```python
from build123d import *

# Parameters (mm, degrees)
SKETCH007_R             = 1.65
PAD005_DEPTH            = 1.6
SKETCH008_R             = 3.55
PAD006_DEPTH            = 16.3
SKETCH009_R             = 1.95
POCKET002_DEPTH         = 12
POCKET003_DEPTH         = 1.6
BODY002_PLACEMENT_ANGLE = 180


with BuildPart() as part:
    # Sketch007 → Pad005 (new body)
    with BuildSketch(Plane.XY):
        with BuildLine():
            Line((-51.5, 40.5), (51.5, 40.5))
            ThreePointArc((54.5, 37.5), (53.62132, 39.62132), (51.5, 40.5))
            Line((54.5, 37.5), (54.5, 14))
            ThreePointArc((54.5, 14), (55.37868, 11.87868), (57.5, 11))
            Line((57.5, 11), (70.5, 11))
            ThreePointArc((73.5, 8), (72.62132, 10.12132), (70.5, 11))
            Line((73.5, 8), (73.5, 3))
            Line((73.5, 3), (75, 3))
            ThreePointArc((75, -3), (78, 0), (75, 3))
            Line((73.5, -3), (75, -3))
            Line((73.5, -3), (73.5, -8))
            ThreePointArc((70.5, -11), (72.62132, -10.12132), (73.5, -8))
            Line((70.5, -11), (57.5, -11))
            ThreePointArc((57.5, -11), (55.37868, -11.87868), (54.5, -14))
            Line((54.5, -14), (54.5, -37.5))
            ThreePointArc((51.5, -40.5), (53.62132, -39.62132), (54.5, -37.5))
            Line((51.5, -40.5), (-51.5, -40.5))
            ThreePointArc((-54.5, -37.5), (-53.62132, -39.62132), (-51.5, -40.5))
            Line((-54.5, -37.5), (-54.5, 37.5))
            ThreePointArc((-51.5, 40.5), (-53.62132, 39.62132), (-54.5, 37.5))
        make_face()
        with Locations((75, 0)):
            Circle(SKETCH007_R, mode=Mode.SUBTRACT)
    extrude(amount=PAD005_DEPTH)

    # Sketch008 → Pad006 (join)
    with BuildSketch(Plane.XY):
        with Locations((-49.75, 35.75)):
            Circle(SKETCH008_R)
        with Locations((-9.75, 35.75)):
            Circle(SKETCH008_R)
        with Locations((9.75, 35.75)):
            Circle(SKETCH008_R)
        with Locations((49.75, 35.75)):
            Circle(SKETCH008_R)
        with Locations((49.75, -35.75)):
            Circle(SKETCH008_R)
        with Locations((9.75, -35.75)):
            Circle(SKETCH008_R)
        with Locations((-9.75, -35.75)):
            Circle(SKETCH008_R)
        with Locations((-49.75, -35.75)):
            Circle(SKETCH008_R)
    extrude(amount=PAD006_DEPTH)

    # Sketch009 (on DatumPlane) → Pocket002 (cut)
    with BuildSketch(Plane.XY.offset(16.3)):
        with Locations((-49.75, 35.75)):
            Circle(SKETCH009_R)
        with Locations((-9.75, 35.75)):
            Circle(SKETCH009_R)
        with Locations((9.75, 35.75)):
            Circle(SKETCH009_R)
        with Locations((49.75, 35.75)):
            Circle(SKETCH009_R)
        with Locations((-49.75, -35.75)):
            Circle(SKETCH009_R)
        with Locations((-9.75, -35.75)):
            Circle(SKETCH009_R)
        with Locations((9.75, -35.75)):
            Circle(SKETCH009_R)
        with Locations((49.75, -35.75)):
            Circle(SKETCH009_R)
    extrude(amount=-POCKET002_DEPTH, mode=Mode.SUBTRACT)

    # Sketch011 → Pocket003 (cut)
    with BuildSketch(Plane.XY):
        with BuildLine():
            ThreePointArc((-25, 5), (-30, 0), (-25, -5))
            Line((-25, -5), (25, -5))
            ThreePointArc((25, -5), (30, 0), (25, 5))
            Line((25, 5), (-25, 5))
        make_face()
    extrude(amount=POCKET003_DEPTH, mode=Mode.SUBTRACT)


with BuildPart() as part_1:
    # Body002 placement: moved
    add(part.part.moved(Location((0, 0, 38))).rotate(Axis((0, 0, 38), (1, 0, 0)), BODY002_PLACEMENT_ANGLE))


solid = part_1.part
```
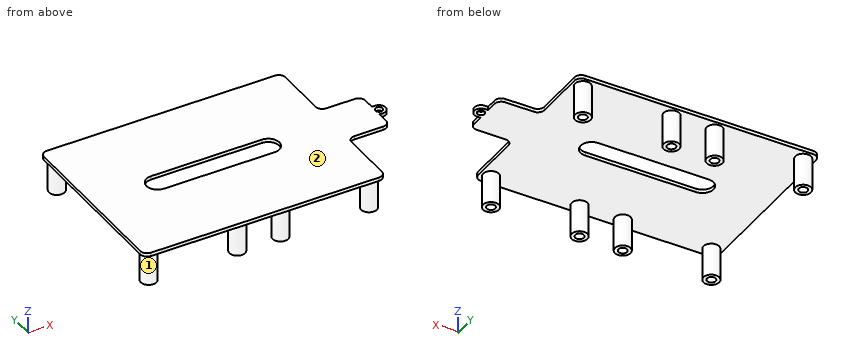
Part model, mm, in its own coordinate system. Face numbers are marked on the shaded views. Give positions to 0.01 mm unless a question says otherwise; leave off trailing zeros. Order: outer loops, then holes, each group sorted by start corner. A loop starts at its lowest first (then second) coordinate and runs counter-clockwise, first axis right, second up. Notation, with made-up numbers: M 35,-26 L 55,-26 A30 cw 55,4 Z; hole C -24,16.5 d4. An arc over 180 degrees is marked long. Use a Markdown table: item, result. Add a question column.
(1) Drop flat-ended pins along their axis: P1, Ø3, axis at x = -16, z = 33, coming from the +Y side; P2, Ø3.5, axis at x = -9.75, y = 35.75, coming from the -Z side; P3, Ø0.5, axis at y = 22.5, z = 37.5, coming from the +X side; P4, Ø1.5, axis at x = 38, y = 2.5, coming from the -Z side. Give the stop position or say it passes through.
(2) Mould opens along X. For the marked faces 1 and 2 say: +X half, -X half, draft (parallel to the pull), parting line (faces both ways), or undercut.
(3) Saw through at A-A, the plane z = 25.5. Give the number of separate pieces and of enclosed holes in the cut face, and give its area (3 significant figures).
(4) Probe line 1 along Y through (x, z) = (-49.75, 28.5); line 2 along X through (y, z) = (37, 36.25); line 3 along Z through (x, y) = (18, 16). List the from-to ranges inside material, lowest first. Write a range as [from, to].
(5) Saw through at C-C, the plane x = 49.75. Give the cut face in (y, z), and give its area (3 significant figures).
(6) Saw through at D-D, the plane y = 18.5. Give the cut face in (x, z).
(7) Saw through at B-B, the plane x = 20. Give the cut face in (y, z).
Answer key:
| question | item | result |
|---|---|---|
| 1 | P1 | through |
| 1 | P2 | z = 33.7 |
| 1 | P3 | x = 54.5 |
| 1 | P4 | z = 36.4 |
| 2 | face 1 | undercut |
| 2 | face 2 | draft |
| 3 | separate pieces | 8 |
| 3 | enclosed holes | 8 |
| 3 | area | 221 mm^2 |
| 4 | line 1 | [-39.3, -37.7], [-33.8, -32.2], [32.2, 33.8], [37.7, 39.3] |
| 4 | line 2 | [-53.07, -46.43], [-13.07, -6.43], [6.43, 13.07], [46.43, 53.07] |
| 4 | line 3 | [36.4, 38] |
| 5 | outline | M -40.5,36.4 L -39.3,36.4 L -39.3,21.7 L -37.7,21.7 L -37.7,33.7 L -33.8,33.7 L -33.8,21.7 L -32.2,21.7 L -32.2,36.4 L 32.2,36.4 L 32.2,21.7 L 33.8,21.7 L 33.8,33.7 L 37.7,33.7 L 37.7,21.7 L 39.3,21.7 L 39.3,36.4 L 40.5,36.4 L 40.5,38 L -40.5,38 Z |
| 5 | area | 245 mm^2 |
| 6 | outline | M -54.5,36.4 L 54.5,36.4 L 54.5,38 L -54.5,38 Z |
| 7 | outline | M -40.5,36.4 L -5,36.4 L -5,38 L -40.5,38 Z; M 5,36.4 L 40.5,36.4 L 40.5,38 L 5,38 Z |
